Autodesk Inventor part; units mm, degrees
ref_plane "YZ Plane" through (0, 0, 0) normal (1, 0, 0) x (0, 1, 0)
ref_plane "XZ Plane" through (0, 0, 0) normal (0, 1, 0) x (-1, 0, 0)
ref_plane "XY Plane" through (0, 0, 0) normal (0, 0, 1) x (1, 0, 0)
sketch "Sketch1" plane through (0, 0, 0) normal (0, 0, 1) x (1, 0, 0)
  line L0 (-204, -167.1829) -> (204, -167.1829) construction
  line L1 (204, -167.1829) -> (204, 115) construction
  line L2 (204, 115) -> (-204, 115) construction
  line L3 (-204, 115) -> (-204, -167.1829) construction
  line L4 (-214, -177.1829) -> (214, -177.1829)
  line L5 (214, -177.1829) -> (214, 125)
  line L6 (214, 125) -> (-214, 125)
  line L7 (-214, 125) -> (-214, -177.1829)
  line L8 (-244, -177.1829) -> (244, -177.1829)
  line L9 (244, -177.1829) -> (244, 175)
  line L10 (244, 175) -> (-244, 175)
  line L11 (-244, 175) -> (-244, -177.1829)
  point P0 (0, 0)
  dimension "d0" = 10
  dimension "d1" = 30
  dimension "d2" = 30
  dimension "d3" = 50
extrude "Extrusion1" add sketch "Sketch1" along normal blind 5 contours L8 L11 L10 L9 L5 L6 L7
sketch "Sketch2" plane through (0, 0, 5) normal (0, 0, 1) x (1, 0, 0)
  line L0 (-214, -177.1829) -> (-214, 125)
  line L1 (-214, 125) -> (214, 125)
  line L2 (214, 125) -> (214, -177.1829)
  line L3 (214, -177.1829) -> (244, -177.1829)
  line L4 (244, -177.1829) -> (244, 175)
  line L5 (244, 175) -> (-244, 175)
  line L6 (-244, 175) -> (-244, -177.1829)
  line L7 (-244, -177.1829) -> (-214, -177.1829)
  line L8 (213.2, 124.2) -> (-213.2, 124.2)
  line L9 (-213.2, 124.2) -> (-213.2, -176.3829)
  line L10 (-244, -177.9829) -> (-244.8, -177.9829)
  line L11 (-244.8, -177.9829) -> (-244.8, 175.8)
  line L12 (-244.8, 175.8) -> (244.8, 175.8)
  line L13 (244.8, 175.8) -> (244.8, -177.9829)
  line L14 (244.8, -177.9829) -> (213.2, -177.9829)
  line L15 (214, 125) -> (214, -177.1829)
  line L16 (-244, -177.1829) -> (-214, -177.1829)
  line L17 (213.2, -177.1829) -> (-214, -177.1829)
  line L18 (213.2, -176.3829) -> (-213.2, -176.3829)
  line L19 (213.2, -177.1829) -> (214, -177.1829)
  line L20 (213.2, -177.9829) -> (213.2, -177.1829)
  line L21 (213.2, -176.3829) -> (213.2, 124.2)
  point P0 (0, 0)
  dimension "d6" = 0.8
  dimension "d7" = 0.8
extrude "Extrusion2" add sketch "Sketch2" against normal blind 300 contours L0 L1 L2 L19 L17
sketch "Sketch3" plane through (0, 0, 5) normal (0, 0, 1) x (1, 0, 0)
  line L0 (-213.2, -176.3829) -> (-213.2, 124.2)
  line L1 (-213.2, 124.2) -> (213.2, 124.2)
  line L2 (213.2, 124.2) -> (213.2, -176.3829)
  line L3 (213.2, -176.3829) -> (-213.2, -176.3829)
  line L4 (-244, -177.1829) -> (244, -177.1829)
  line L5 (244, -177.1829) -> (244, 175)
  line L6 (244, 175) -> (-244, 175)
  line L7 (-244, 175) -> (-244, -177.1829)
  line L8 (243.2, -176.3829) -> (-243.2, -176.3829)
  line L9 (-243.2, -176.3829) -> (-243.2, 174.2)
  line L10 (-243.2, 174.2) -> (243.2, 174.2)
  line L11 (243.2, 174.2) -> (243.2, -176.3829)
  point P0 (0, 0)
  dimension "d10" = 0.8
extrude "Extrusion3" add sketch "Sketch3" along normal blind 30
sketch "Sketch5" plane through (0, 0, -295) normal (0, 0, -1) x (-1, 0, 0)
  line L0 (213.2, 124.2) -> (213.2, -176.3829)
  line L1 (213.2, -176.3829) -> (-213.2, -176.3829)
  line L2 (-213.2, -176.3829) -> (-213.2, 124.2)
  line L3 (-213.2, 124.2) -> (213.2, 124.2)
  line L4 (-214, -177.1829) -> (214, -177.1829)
  line L5 (214, -177.1829) -> (214, 125)
  line L6 (214, 125) -> (-214, 125)
  line L7 (-214, 125) -> (-214, -177.1829)
  point P0 (0, 0)
extrude "Extrusion5" add sketch "Sketch5" along normal blind 0.8 contours L0 L1 L2 L3 | L7 L6 L5 L4
sketch "Sketch7" plane through (214, -177.1829, 0) normal (0, -1, 0) x (1, 0, 0)
  line L0 (0, 0) -> (30, 0)
  line L1 (30, 0) -> (30, 35)
  line L2 (-458, 35) -> (30, 35)
  line L3 (-458, 0) -> (-458, 35)
  line L4 (-458, 0) -> (-428, 0)
  line L5 (-428, 0) -> (-428, -295.8)
  line L6 (0, -295.8) -> (-428, -295.8)
  line L7 (0, 0) -> (0, -295.8)
  point P0 (-214, 0)
extrude "Extrusion7" add sketch "Sketch7" along normal blind 4.2
sketch "Sketch10" plane through (-214, 125, 0) normal (0, 1, 0) x (1, 0, 0)
  line L0 (428, 0) -> (0, 0)
  line L1 (428, 0) -> (428, 295.8)
  line L2 (0, 295.8) -> (428, 295.8)
  line L3 (0, 0) -> (0, 295.8)
  point P0 (214, 0)
extrude "Extrusion10" add sketch "Sketch10" along normal blind 4.2
sketch "Sketch12" plane through (0, 0, 5) normal (0, 0, 1) x (1, 0, 0)
  line L0 (214, 129.2) -> (-214, 129.2)
  line L1 (-214, 129.2) -> (214, 129.2)
  line L2 (214, 129.2) -> (214, 159.2)
  line L3 (214, 159.2) -> (-214, 159.2)
  line L4 (-214, 159.2) -> (-214, 129.2)
  point P0 (0, 0)
  dimension "d35" = 30
extrude "Extrusion12" cut sketch "Sketch12" against normal through all
sketch "Sketch13" plane through (-214, 129.2, 0) normal (0, 1, 0) x (1, 0, 0)
  line L0 (428, -5) -> (428, 0)
  line L1 (0, -5) -> (0, 0)
  line L2 (214, -68.5291) -> (214, 358.2531) construction
  line L3 (428, 0) -> (235.9552, 130)
  line L4 (192.0448, 130) -> (0, 0)
  line L5 (-29.2, -5) -> (0.8, -5)
  line L6 (428, 0) -> (458, 0)
  line L7 (235.9552, 130) -> (192.0448, 130)
  line L8 (-0.8, 0.4245) -> (191.7995, 130.8)
  line L9 (191.7995, 130.8) -> (236.2005, 130.8)
  line L10 (236.2005, 130.8) -> (428.4485, 0.6625)
  line L11 (428.4485, 0.6625) -> (429.4271, 0)
  line L12 (-0.8, 0.4245) -> (-1.4271, 0)
  line L13 (429.4271, 0) -> (428, 0)
  line L14 (0, 0) -> (0, 295.8)
  line L15 (0, 0) -> (-1.4271, 0)
  point P0 (214, 0)
  point P1 (427.2, -5)
  dimension "d41" = 0.8
extrude "Extrusion13" add sketch "Sketch13" along normal up to surface (30 mm away)
sketch "Sketch14" plane through (-22.2005, 159.2, -130.8) normal (0, 1, 0) x (1, 0, 0)
  line L0 (236.2005, -130.8) -> (44.1556, -0.8)
  line L1 (237.6276, -130.8) -> (236.2005, -130.8)
  line L2 (44.401, 0) -> (237.6276, -130.8)
  line L3 (0, 0) -> (44.401, 0)
  line L4 (-193.2266, -130.8) -> (0, 0)
  line L5 (-191.7995, -130.8) -> (-193.2266, -130.8)
  line L6 (0.2453, -0.8) -> (-191.7995, -130.8)
  line L7 (44.1556, -0.8) -> (0.2453, -0.8)
  line L8 (236.2005, -130.8) -> (44.1556, -0.8)
  line L9 (236.2005, -130.8) -> (-191.7995, -130.8)
  line L10 (236.2005, -130.8) -> (-191.7995, -130.8)
  point P0 (22.2005, -130.8)
extrude "Extrusion14" add sketch "Sketch14" along normal blind 0.8
sketch "Sketch15" plane through (-22.2005, 160, -130.8) normal (0, 1, 0) x (1, 0, 0)
  point P0 (22.2005, -130.8)
sketch "Sketch16" plane through (22.2005, 129.2, -130.8) normal (0, 0, -1) x (-1, 0, 0)
  circle A0 centre (22.2005, 18.5941) radius 7.5
  point P0 (22.2005, -129.2)
  dimension "d46" = 15
extrude "Extrusion15" cut sketch "Sketch16" against normal blind 0.8
sketch "Sketch17" plane through (22.2005, 129.2, -130.8) normal (0, 0, -1) x (-1, 0, 0)
  circle A0 centre (22.2005, 18.5941) radius 7.5
  circle A1 centre (22.2005, 18.5941) radius 6.5
  point P0 (22.2005, -129.2)
  dimension "d49" = 1
extrude "Extrusion16" add sketch "Sketch17" along normal blind 20
sketch "Sketch18" plane through (214, -181.3829, 0) normal (0, -1, 0) x (1, 0, 0)
  circle A0 centre (-408, 17.5) radius 7.5
  circle A1 centre (-358, 17.5) radius 7.5
  line L0 (-458, 35) -> (-458, 0)
  point P0 (-214, 0)
  dimension "d52" = 15
  dimension "d53" = 15
  dimension "d54" = 50
  dimension "d55" = 50
extrude "Extrusion17" cut sketch "Sketch18" against normal blind 20
sketch "Sketch19" plane through (-243.2, -176.3829, 5) normal (0, 1, 0) x (1, 0, 0)
  circle A0 centre (99.2, -12.5) radius 7.5
  circle A1 centre (49.2, -12.5) radius 7.5
  circle A2 centre (99.2, -12.5) radius 6.5
  circle A3 centre (49.2, -12.5) radius 6.5
  point P0 (243.2, 5)
  dimension "d58" = 1
  dimension "d59" = 1
extrude "Extrusion18" add sketch "Sketch19" against normal blind 20
sketch "Sketch20" plane through (0, 147.7941, -130.8) normal (0, 0, 1) x (1, 0, 0)
  circle A0 centre (0, 0) radius 6.5
  circle A1 centre (0, 0) radius 7.5
  point P0 (0, -147.7941)
extrude "Extrusion19" add sketch "Sketch20" along normal up to surface (0.8 mm away)
sketch "Sketch21" plane through (-214, -181.3829, -295.8) normal (-1, 0, 0) x (0, 0, 1)
  line L0 (300.8, 305.5829) -> (0.8, 305.5829)
  line L1 (0.8, 305.5829) -> (0.8, 5)
  circle A0 centre (8.3, 298.0829) radius 7.5
  point P0 (295.8, 181.3829)
  dimension "d64" = 15
extrude "Extrusion20" cut sketch "Sketch21" against normal blind 20 contours A0
sketch "Sketch22" plane through (-213.2, -176.3829, 5) normal (1, 0, 0) x (0, 0, -1)
  circle A0 centre (292.5, 293.0829) radius 7.5
  circle A1 centre (292.5, 293.0829) radius 6.5
  point P0 (5, 176.3829)
  dimension "d67" = 1
extrude "Extrusion21" add sketch "Sketch22" against normal blind 20
properties part number "Tank2"
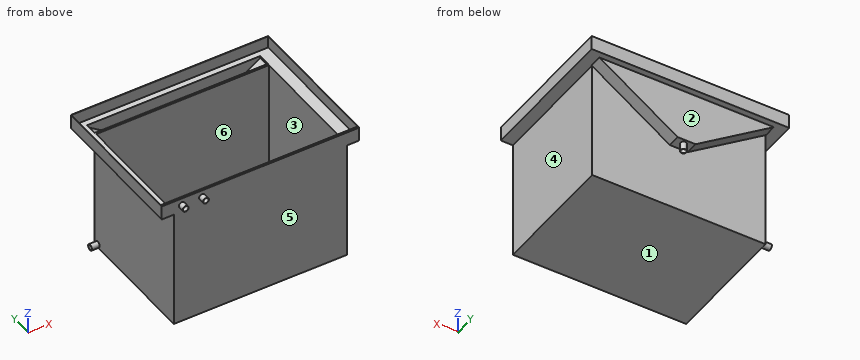
Read the model definition and answer for the solid it produces. Units are mm, in the model's axes. Face numbers are marked on the shaded views. A direction names the side the tool comes from. Coordinates: 2 decimals unless noted, no trailing zeros. Loops run counter-clockwise (first coordinate to the right, second up) from the corner with the lowest first, then second, coordinate; pieces in that order, holes last.
Q1. The part is cut by section D-D on y = 18. Write down the section's boundary in (x, z).
Q2. The mould has two halves that part along Y. Classify the marked faces 3, 4, 5 and 6: +Y half, -Y half, draft (parallel to the pull), parting line (faces both ways), or undercut.
Q3. Which of the six approach directions +Z, -Z, +X, -X, +Y, -Y give full straight-line access (tool end or side, diameter ignored) to the marked faces 1 and 2?
Q4. Consider probe 1 along Y at (x, z) = (-55, -50.5); probe 2 along X at (y, z) = (-180, 17); probe 3 along Y at (x, z) = (61, -269). Determine where each line is inside the solid, lowest interval first.
Q5. The part is cut by section C-C on y = 116.7. Write down the section's boundary in (x, z).
Q6. The part is cut by section A-A on x = 0. Write down the section's boundary in (y, z), and give its area (3 significant figures).
Q7. Each of these flat-tipped pins is pushed along its axis until it touches: pin 1 Ø6 at (y, z) = (-116, -217.5) entering from -X; pin 2 Ø12 at (x, z) = (-182, -213) entering from +Y; pin 3 Ø16.5 at (y, z) = (115, -285.5) entering from -X. Where does it stop, or does it pass through?
Q8. The part is cut by section B-B on z = 17.5. Write down the section's boundary in (x, y).
Results below:
1. outline: (-244, 0) - (-214, 0) - (-214, -295.8) - (214, -295.8) - (214, 0) - (244, 0) - (244, 35) - (243.2, 35) - (243.2, 5) - (213.2, 5) - (213.2, -295) - (-213.2, -295) - (-213.2, 5) - (-243.2, 5) - (-243.2, 35) - (-244, 35) - close
2. face 3: undercut
2. face 4: draft
2. face 5: -Y half
2. face 6: undercut
3. face 1: -Z, +X, -X, +Y, -Y
3. face 2: -Z, +X, -X, +Y
4. probe 1: y = -181.38 to -176.38, 124.2 to 129.2, 159.2 to 160
4. probe 2: x = -244 to -200.48, -187.52 to -150.48, -137.52 to 244
4. probe 3: y = -181.38 to -176.38, 124.2 to 129.2
5. outline: (-244, 0) - (-214, 0) - (-214, -280) - (-233.2, -280) - (-233.2, -281) - (-213.2, -281) - (-213.2, 5) - (-243.2, 5) - (-243.2, 35) - (-244, 35) - close; (-233.2, -295) - (-214, -295) - (-214, -295.8) - (214, -295.8) - (214, 0) - (244, 0) - (244, 35) - (243.2, 35) - (243.2, 5) - (213.2, 5) - (213.2, -295) - (-213.2, -295) - (-213.2, -294) - (-233.2, -294) - close
6. outline: (-181.38, -295.8) - (129.2, -295.8) - (129.2, -130.8) - (140.29, -130.8) - (140.29, -150.8) - (141.29, -150.8) - (141.29, -130) - (129.2, -130) - (129.2, 5) - (124.2, 5) - (124.2, -295) - (-176.38, -295) - (-176.38, 35) - (-181.38, 35) - close; (154.29, -150.8) - (155.29, -150.8) - (155.29, -130.8) - (160, -130.8) - (160, 0) - (175, 0) - (175, 35) - (174.2, 35) - (174.2, 5) - (159.2, 5) - (159.2, -130) - (154.29, -130) - close
6. area: 3,660 mm2
7. pin 1: stops at x = -214
7. pin 2: stops at y = 129.2
7. pin 3: stops at x = -233.2
8. outline: (-244, -181.38) - (-201.5, -181.38) - (-201.5, -196.38) - (-200.5, -196.38) - (-200.5, -176.38) - (-243.2, -176.38) - (-243.2, 174.2) - (243.2, 174.2) - (243.2, -176.38) - (-137.5, -176.38) - (-137.5, -196.38) - (-136.5, -196.38) - (-136.5, -181.38) - (244, -181.38) - (244, 175) - (-244, 175) - close; (-187.5, -196.38) - (-186.5, -196.38) - (-186.5, -181.38) - (-151.5, -181.38) - (-151.5, -196.38) - (-150.5, -196.38) - (-150.5, -176.38) - (-187.5, -176.38) - close
